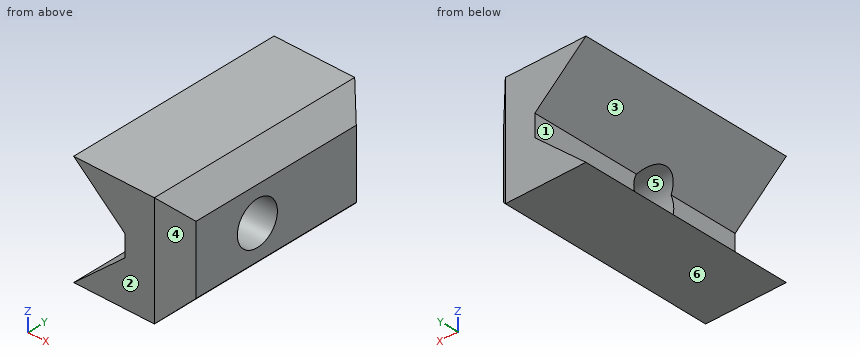
Autodesk Inventor part; units mm, degrees
ref_plane "YZ Plane" through (0, 0, 0) normal (1, 0, 0) x (0, 1, 0)
ref_plane "XZ Plane" through (0, 0, 0) normal (0, 1, 0) x (-1, 0, 0)
ref_plane "XY Plane" through (0, 0, 0) normal (0, 0, 1) x (1, 0, 0)
sketch "Sketch1" plane through (0, 0, 0) normal (0, 1, 0) x (-1, 0, 0)
  line L0 (4.725, 5.15) -> (-4.725, 5.15)
  line L1 (-4.725, 5.15) -> (-4.725, -5.15)
  line L2 (-4.725, -5.15) -> (4.725, -5.15)
  line L3 (4.725, 5.15) -> (-4.725, -5.15) construction
  line L4 (-4.725, 5.15) -> (4.725, -5.15) construction
  line L5 (0, 0) -> (0, -1)
  line L6 (0, 0) -> (0, 1)
  line L7 (0, -1) -> (4.725, -5.15)
  line L8 (0, 1) -> (4.725, 5.15)
  dimension "d0" = 9.45
  dimension "d1" = 10.3
  dimension "d2" = 1
  dimension "d3" = 1
extrude "Extrusion1" add sketch "Sketch1" along normal blind 20
sketch "Sketch2" plane through (4.725, 0, 5.15) normal (1, 0, 0) x (0, 0, -1)
  line L0 (10.3, 0) -> (0, 0) construction
  line L1 (10.3, 0) -> (10.3, 20) construction
  line L2 (0, 20) -> (10.3, 20) construction
  line L3 (0, 0) -> (0, 20) construction
  point P0 (5.15, 0)
  point P1 (5.15, 8.125)
hole "Hole1" at (4.725, 8.125, 0) direction (-1, 0, 0) diameter 4 end through all
chamfer "Chamfer1" distance 2 angle 45 4 edges at (4.725, 10, 5.15) (4.725, 0, 0) (4.725, 10, -5.15) (4.725, 20, 0)
properties part number "nut_part"
Here's how the part is built. I have some questions about the finished solid (model axes, mm). Face numbers are marked on the shaded views. A direction names the side the tool comes from. Round coordinates to 2 decimals unless told otherwise and drop trailing zeros. Order: outer loops, then holes, each group sorted by start corner. A loop starts at its lowest first (then second) coordinate and runs counter-clockwise, first axis right, second up. Notation, with made-up numbers: (26, -20.5) -> (64, -20.5) arc R19 cw to (64, -9.5) -> close; hole circle Ø9 at (-15, 89). An arc over 180 degrees is marked (long way). Return JSON: item names as keys, results as strings.
Q1. If we section it at D-D on x = 1.25: List the corners of the cut face in (y, z) for me (3 decimals), plus the area to 3 significant figures.
Filled sheet:
{"outline": "(0, -5.15) -> (20, -5.15) -> (20, 5.15) -> (0, 5.15) -> close; hole circle Ø4 at (8.125, 0)", "area": "193 mm^2"}
Q2. I need wall thicknesses on line 1 along Y through (x, z) = (2, 0) (3 decimals); line 2 along Z through (x, y) = (-4, 2.5); line 3 along Z through (x, y) = (-3.25, 7.5). Which ranges of each line are inside material? Lowest first, please. Write a range as from..to.
Filled sheet:
{"line 1": "y = 0..6.125, 10.125..20", "line 2": "z = -5.15..-4.51, 4.51..5.15", "line 3": "z = -5.15..-3.85, 3.85..5.15"}
Q3. If we section it at B-B on z = 0: List the corners of the cut face in (x, y) for me (3 decimals), plus the area to 3 significant figures.
Filled sheet:
{"outline": "(0, 0) -> (2.725, 0) -> (4.725, 2) -> (4.725, 6.125) -> (0, 6.125) -> close; (0, 10.125) -> (4.725, 10.125) -> (4.725, 18) -> (2.725, 20) -> (0, 20) -> close", "area": "71.6 mm^2"}
Q4. For pin 1 Ø5 at (y, z) = (8.125, 0) entering from -X; pin 2 Ø0.6 at (y, z) = (4.5, 0.5) entering from -X; pin 3 Ø6 at (y, z) = (9, 2) entering from -X, each with a flat end and sliding along its axis, tell me the tip position at first contact or that it passes through.
Filled sheet:
{"pin 1": "stops at x = -1.71", "pin 2": "stops at x = 0", "pin 3": "stops at x = -4.55"}
Q5. Which directions (+Z, -Z, +X, -X, +Y, -Y) give clear straight access to the entire face, cutting with the end or side of a thin tool? Please do the marked faces 1 and 2.
Filled sheet:
{"face 1": "-X, +Y, -Y", "face 2": "+Z, -Z, +X, -X, -Y"}
Q6. If we mould it in two halves opening along Z, with no side actions, what happens to the marked faces 3, 4, 5 and 6? For each: released by +Z, released by -Z, zero draft, split by the parting line, or undercut.
Filled sheet:
{"face 3": "undercut", "face 4": "zero draft", "face 5": "undercut", "face 6": "released by -Z"}
Q7. If we section it at C-C on x = -2.75: List the corners of the cut face in (y, z) for me, plus the area to 3 significant figures.
Filled sheet:
{"outline": "(0, -5.15) -> (20, -5.15) -> (20, -3.42) -> (0, -3.42) -> close; (0, 3.42) -> (20, 3.42) -> (20, 5.15) -> (0, 5.15) -> close", "area": "69.4 mm^2"}
Q8. If we section it at A-A on y = 16.5: List the corners of the cut face in (x, z) for me (3 decimals), plus the area to 3 significant figures.
Filled sheet:
{"outline": "(-4.725, -5.15) -> (2.725, -5.15) -> (4.725, -3.15) -> (4.725, 3.15) -> (2.725, 5.15) -> (-4.725, 5.15) -> (0, 1) -> (0, -1) -> close", "area": "64.3 mm^2"}
